from build123d import *

# Parameters (mm, degrees)
SKETCH_1_W      = 270
SKETCH_1_H      = 56
EXTRUDE_1_DEPTH = 8


with BuildPart() as part:
    # Эскиз1 → Бобышка-Вытянуть1 (new body)
    with BuildSketch(Plane(origin=(0, 0, 0), x_dir=(1, 0, 0), z_dir=(0, 1, 0))):
        Polygon((320, 170), (320, 60), (225, 0), (0, 0), (0, 170), align=None)
        with Locations((165, 118)):
            Rectangle(SKETCH_1_W, SKETCH_1_H, mode=Mode.SUBTRACT)
    extrude(amount=EXTRUDE_1_DEPTH)


solid = part.part
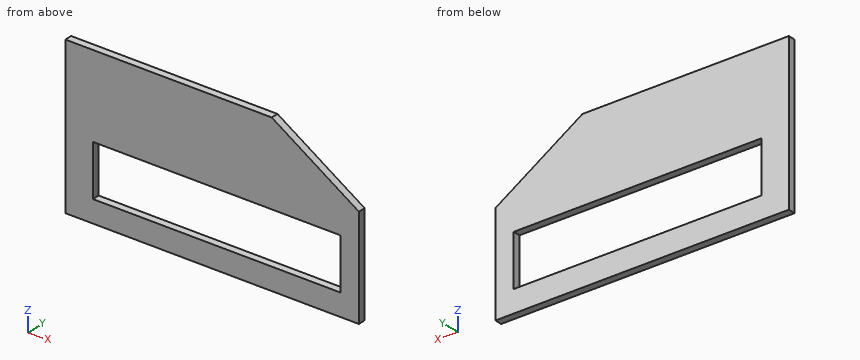
Here's how the part is built. I have some questions about the finished solid (model axes, mm). Coordinates: 2 decimals unless noted, no trailing zeros. Write each loop counter-clockwise with the first axis right and the second up, starting at its lowest first coordinate (ties: lowest second). Pieces come first, ordered by that corner, then holes.
1) If we section it at D-D (z = -19.5): List the corners of the cut face in (x, y) for me (3 decimals).
Filled in:
outline: (0, 0) - (255.875, 0) - (255.875, 8) - (0, 8) - close
2) If we section it at A-A (z = -130): List the corners of the cut face in (x, y) for me, plus the area to 3 significant figures.
Filled in:
outline: (0, 0) - (30, 0) - (30, 8) - (0, 8) - close; (300, 0) - (320, 0) - (320, 8) - (300, 8) - close
area: 400 mm2
3) If I drill on line 1 (Z direction, x = 40.5, y = 7); line 2 (X direction, y = 5.25, z = -140); line 3 (Z direction, x = 288.5, y = 4), over which ranges is the centre line in solid material (lowest first)?
Filled in:
line 1: z = -170 to -146, -90 to 0
line 2: x = 0 to 30, 300 to 320
line 3: z = -170 to -146, -90 to -40.11
4) If we section it at C-C (x = 44.5): List the corners of the cut face in (y, z) for me, plus the area to 3 significant figures.
Filled in:
outline: (0, -170) - (8, -170) - (8, -146) - (0, -146) - close; (0, -90) - (8, -90) - (8, 0) - (0, 0) - close
area: 912 mm2
5) If we section it at B-B (y = 1.75): List the corners of the cut face in (x, z) for me.
Filled in:
outline: (0, -170) - (320, -170) - (320, -60) - (225, 0) - (0, 0) - close; hole (30, -146) - (300, -146) - (300, -90) - (30, -90) - close
